Verification items for this drawing (mm, ordinates from the low corner). A direction names the side the tool comes from. Give positions to 0.01 mm unless a question says otherwise; leave off trailing zeros. Loops run counter-clockwise (first coordinate to the right, second up) from the corner with the lowest first, then second, coordinate; pieces in that order, holes last. Notation, with made-up numbers: (8.5, 5.5) -> (14.5, 5.5) arc R24 ccw to (14.5, 37.5) -> close; hole circle Ø9 at (43.25, 6.5). An arc over 180 degrees is marked (long way). Write each question's results on one line, items separated by ' | '. Start each with the question number.
1) Scan lines: line 1 (Y direction, x = 15.5, z = 27); line 2 (Z direction, x = 34, y = 64); line 3 (Y direction, x = 10, z = 106) (1 decimal). Record each from-to range of solid material in increasing order. Write a range as from..to.
2) Draft check along Z on the marked faces 3, 4 and 5. Enter one of: pulls with the +Z half, pulls with the -Z half, needs draft (parallel to the pull), parting line crosses it, or undercut.
3) Sectioned sample at D-D on y = 57. Record the cut outline in (x, z).
4) Set-up check for the marked faces 1 and 2: record each of +Z, -Z, +X, -X, +Y, -Y from which the full face is reachable in a straight line by a thin tool's end or side.
5) Sectioned sample at A-A on y = 47. Record the cut outline in (x, z), then the cut area to 3 significant figures.
6) Sectioned sample at C-C on z = 35. Record the cut outline in (x, y).
7) Sectioned sample at B-B on x = 43. Record the cut outline in (y, z), then the cut area to 3 significant figures.
8) Depth check by flat-ended pin: pin 1 (2 mm diameter, centred on x = 20, y = 60, fed in from -Z); pin 2 (6 mm diameter, centred on x = 13, y = 59, fed in from +Z); pin 3 (5 mm diameter, centred on x = 43.5, z = 105, fed in from -Y). Enter the tip coordinate at first touch or a pass-through.
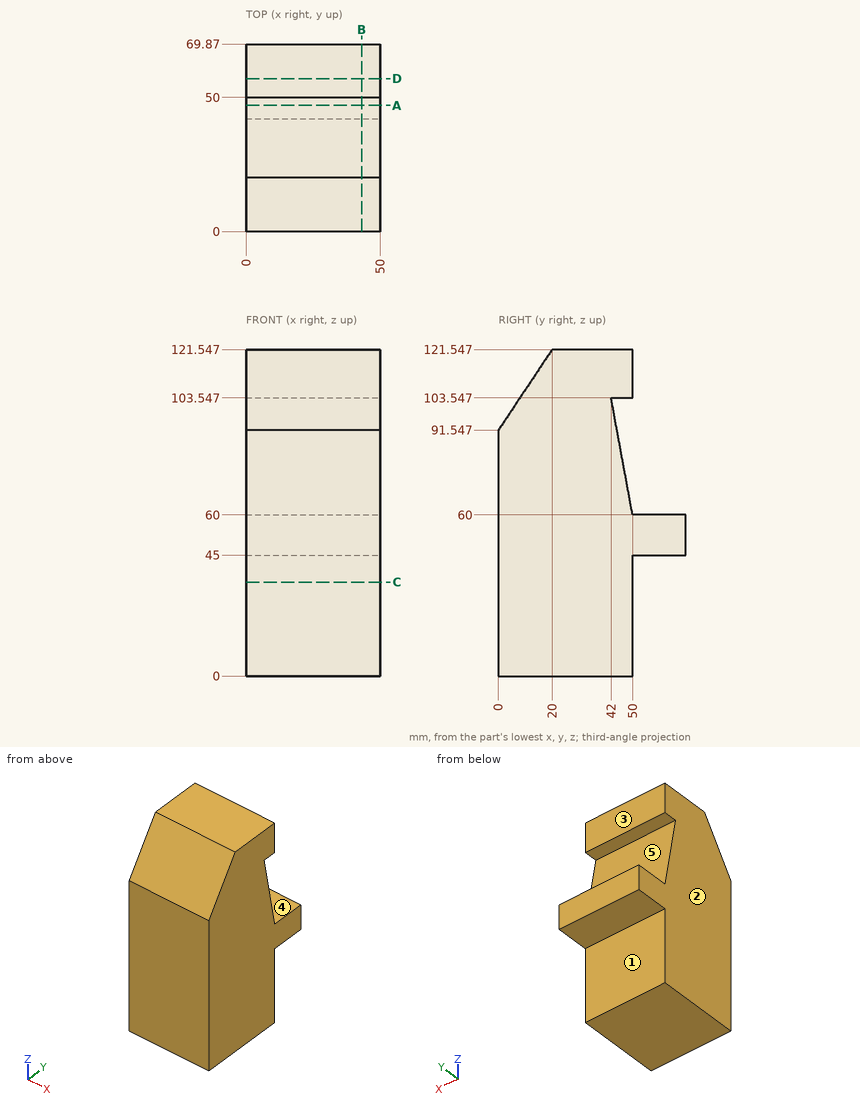
Result:
1) line 1: 0..50 | line 2: 45..60 | line 3: 9.6..50
2) face 3: needs draft | face 4: pulls with the +Z half | face 5: undercut
3) outline: (0, 45) -> (50, 45) -> (50, 60) -> (0, 60) -> close
4) face 1: -Z, +X, -X, +Y | face 2: +Z, -Z, -X, +Y, -Y
5) outline: (0, 0) -> (50, 0) -> (50, 76.33) -> (0, 76.33) -> close; (0, 103.55) -> (50, 103.55) -> (50, 121.55) -> (0, 121.55) -> close | area: 4,720 mm^2
6) outline: (0, 0) -> (50, 0) -> (50, 50) -> (0, 50) -> close
7) outline: (0, 0) -> (50, 0) -> (50, 45) -> (69.87, 45) -> (69.87, 60) -> (50, 60) -> (42, 103.55) -> (50, 103.55) -> (50, 121.55) -> (20, 121.55) -> (0, 91.55) -> close | area: 5,900 mm^2
8) pin 1: z = 45 | pin 2: z = 60 | pin 3: y = 7.3
